Work out the finished part from the listing and answer in its coordinate system (mm). Round coordinates to 2 decimals unless told otherwise and drop trailing zeros. Write each loop counter-clockwise with the first axis right and the second up, starting at its lowest first coordinate (ties: lowest second). Pieces come first, ordered by that corner, then holes. Notation, with made-up numbers: M -23,-8 L 34,-8 A13 ccw 34,0 Z; hole C 36.5,31.5 d3. An arc over 180 degrees is marked long. One line per item, written item: value. Start each with the question number.
Q1. Consider probe 1 along Z at (x, y) = (51.5, 7); probe 2 along Z at (x, y) = (48, -10); probe 3 along X at (y, z) = (-14.5, -87). Determine where each line is inside the solid, lowest interval first.
Q2. Find section A-A (z = -84). Write down the section's boundary in (x, y).
Q3. The mould has two halves that part along X. Classify faces 1 (the flat face through (46, 0, -140.449)), 2 (the flat face through (58, 4, -141.449)), 3 (the cylindrical face through (50.989, -2.174, -140.956)), 4 (the cylindrical face through (62.184, 11.002, -102.349)): released by +X, released by -X, zero draft, split by the parting line, or undercut.
Q4. Given pin 1 Ø0.8 at (x, z) = (51.5, -141) entering from -Y; pin 2 Ø2 at (y, z) = (-7, -121) entering from -X; pin 3 Ø0.8 at (x, z) = (48, -140.5) entering from +Y, each flat-ended and moving along its own axis, determine where each tip first touches the part or whether it passes through.
from build123d import *

# Parameters (mm, degrees)
FILLET1_R           = 10
SKETCH3_R           = 10.606635926
CUT_EXTRUDE1_DEPTH  = 1
FILLET2_R           = 1
BOSS_EXTRUDE1_DEPTH = 1
SKETCH5_R           = 1.357466481
CUT_EXTRUDE2_DEPTH  = 1


# Some blends are built 0.0001 mm under size
with BuildPart() as part:
    # Sketch2 → Revolve1 (revolve)
    with BuildSketch(Plane(origin=(0, 0, 0), x_dir=(1, 0, 0), z_dir=(0, 1, 0))):
        with BuildLine():
            Line((47.835513338, 141.44915936), (36.680360926, 141.44915936))
            Line((36.680360926, 141.44915936), (36.680360926, 139.695253367))
            Line((36.680360926, 139.695253367), (29.754604349, 132.769496791))
            Line((29.754604349, 132.769496791), (29.754604349, 72.768696414))
            ThreePointArc((29.754604349, 72.768696414), (31.416045745, 69.893157133), (34.624175548, 69.034660285))
            Line((34.624175548, 69.034660285), (47.835513338, 69.034660285))
            Line((47.835513338, 69.034660285), (47.835513338, 141.44915936))
        make_face()
    revolve(axis=Axis((47.835513338, 0, -141.44915936), (0, 0, 1)))

    # Fillet1
    # the kernel refuses this fillet: 10 mm, written as the material it adds along each edge
    with BuildSketch(Plane(origin=(47.835513338, 0, -139.695253367), x_dir=(-1, 0, 0), z_dir=(0, 1, 0))) as fillet1_piece_1:
        with BuildLine():
            CenterArc((20.759977074, -4.537310962), FILLET1_R, 135, 28.838814676)
            Line((13.688909262, 2.533756849), (13.547487906, 2.675178206))
            Line((13.547487906, 2.675178206), (11.013731056, 0.141421356))
            Line((11.013731056, 0.141421356), (10.955152412, 0))
            ThreePointArc((10.955152412, 0), (10.955152412, -0.876952996), (10.963055919, -1.698237893))
            Line((10.963055919, -1.698237893), (11.155152412, -1.753905993))
        make_face()
    revolve(axis=Axis((47.835513338, 0, -139.695253367), (0, 0, 1)))

    # Sketch3 → Cut-Extrude1 (cut)
    with BuildSketch(Plane(origin=(0, 0, -141.44915936), x_dir=(-1, 0, 0), z_dir=(0, 0, -1))):
        with Locations((-47.835513338, 0)):
            Circle(SKETCH3_R)
    extrude(amount=-CUT_EXTRUDE1_DEPTH, mode=Mode.SUBTRACT)

    # Fillet2
    fillet2_edges = [part.edges().sort_by_distance(p)[0] for p in [
        (58.442149264, 0, -140.44915936),
    ]]
    fillet(fillet2_edges, radius=FILLET2_R - 0.0001)  # a hair under: the kernel refuses the full size

    # Sketch4 → Boss-Extrude1 (add)
    with BuildSketch(Plane(origin=(0, 0, -140.44915936), x_dir=(-1, 0, 0), z_dir=(0, 0, -1))):
        Polygon((-53.244860259, -2.527826931), (-53.930670857, -1.191951097), (-53.930670857, 0), (-53.39712733, 0.986747489), (-52.726937837, 0.986747489), (-52.00416544, 0.986747489), (-51.028572962, 1.090883539), (-49.975577249, 1.090883539), (-48.95869179, 1.090883539), (-48.872046113, 1.251128017), (-47.819832156, 1.251128017), (-47.746875393, 1.211679618), (-47.373781513, 0.484938009), (-47.166149857, -0.344127446), (-47.166149857, -1.087168011), (-47.560328453, -1.81617084), (-47.945127508, -2.527826931), (-48.375815512, -2.527826931), (-49.1103871, -2.527826931), (-49.975577249, -2.527826931), (-50.676613698, -2.703394925), (-51.754528733, -2.703394925), (-52.341537829, -2.85040584), align=None)
    extrude(amount=BOSS_EXTRUDE1_DEPTH)

    # Sketch5 → Cut-Extrude2 (cut)
    with BuildSketch(Plane(origin=(0, 0, -141.44915936), x_dir=(-1, 0, 0), z_dir=(0, 0, -1))):
        with Locations((-51.615276347, -0.969807614)):
            Circle(SKETCH5_R)
    extrude(amount=-CUT_EXTRUDE2_DEPTH, mode=Mode.SUBTRACT)


solid = part.part
The answers:
1. probe 1: -140.45 to -69.03
1. probe 2: -140.53 to -69.03
1. probe 3: 37.03 to 58.64
2. outline: C 47.84,0 d36.16
3. face 1: undercut
3. face 2: zero draft
3. face 3: undercut
3. face 4: split by the parting line
4. pin 1: y = -10.89
4. pin 2: x = 30.78
4. pin 3: y = 11.65
